Source: CAD feature listing. Evaluate the final solid. Frame: model axes, mm. A direction names the side the tool comes from. Coordinates: 2 decimals unless noted, no trailing zeros. Loops run counter-clockwise (first coordinate to the right, second up) from the corner with the lowest first, then second, coordinate; pieces in that order, holes last. Notation, with made-up numbers: M -10.75,89.5 L 8.25,89.5 A15 cw 8.25,107.5 Z; hole C 17,77.25 d3. An arc over 180 degrees is marked long. One line per question, with ' | ' between items. Start each with the question number.
1. Section query A-A, the plane y = -6.75. Output: boundary loops of the cut face in (x, z), and give its area (3 significant figures).
2. Section query D-D, the plane z = 2.25. Output: boundary loops of the cut face in (x, y).
3. Pin query (flat end, axial travel): P1, Ø6, axis at y = 6, z = -1, coming from the -X side; P2, Ø1.2, axis at x = 143.5, z = -5.5, coming from the +Y side (3 decimals); P3, Ø2, axis at x = 143.5, z = -4.5, coming from the -Y side (3 decimals). Return the tip coordinate at first contact, or that it passes through.
4. Ray query, probe 1 along X at (y, z) = (7.5, -6.5); probe 2 along X at (y, z) = (0.5, -1.25); probe 3 along Y at (x, z) = (3, -4.5). Return the intervals inside material, ascending.
5. Mould query, pull axis X, two halves, no side actions, for faces 1 (the flat face through (-2, -2.375, -5)), 2 (the flat face through (117.25, -4.5, -2.7)), 3 (the flat face through (24.75, 2, 0)), 4 (the flat face through (16.75, -4.5, -2.7)). Classes: pulls with the +X half, pulls with the -X half, needs draft (parallel to the pull), parting line crosses it, or undercut.
6. Section query B-B, the plane z = -4.75. Output: boundary loops of the cut face in (x, y) (3 decimals), and give its area (3 significant figures).
7. Access query for faces 5 (the cylindrical face through (133.508, 4.637, -5.78)), 6 (the flat face through (144, 2.375, -5)), 7 (the flat face through (144, -2.375, -5)), 8 (the cylindrical face through (70.352, 4.637, -5.78)). Directions: +Z, -Z, +X, -X, +Y, -Y. A direction counts if a zero-diameter tool reaches every point of the face in a straight line with its end or side. Return the directions, or none.
8. Section query C-C, the plane y = 0. Output: boundary loops of the cut face in (x, z) (3 decimals).
```python
from build123d import *

# Parameters (mm, degrees)
ESQUISSE5_W        = 4.75
ESQUISSE5_H        = 4.75
BOSS_EXTRU_3_DEPTH = 4
BOSS_EXTRU_4_DEPTH = 4


with BuildPart() as part:
    # Esquisse1 → Révolution1 (revolve)
    with BuildSketch(Plane(origin=(0, 0, 0), x_dir=(1, 0, 0), z_dir=(0, 1, 0))):
        Polygon((0, 0), (0, 4.75), (142, 4.75), (142, 0), (125.25, 0), (125.25, -5), (117.25, -5), (117.25, 0), (24.75, 0), (24.75, -5), (16.75, -5), (16.75, 0), align=None)
    revolve(axis=Axis((0, 0, -4.75), (1, 0, 0)))

    # Esquisse5 → Boss.-Extru.3 (add)
    with BuildSketch(Plane(origin=(142, 0, 0), x_dir=(0, 0, -1), z_dir=(1, 0, 0))):
        with Locations((4.75, 0)):
            Rectangle(ESQUISSE5_W, ESQUISSE5_H)
    extrude(amount=BOSS_EXTRU_3_DEPTH)

    # Esquisse6 → Boss.-Extru.4 (add)
    with BuildSketch(Plane.ZY):
        Polygon((-4.75, 2.375), (-7.125, 2.375), (-7.125, -2.375), (-2.375, -2.375), (-2.375, 2.375), align=None)
    extrude(amount=BOSS_EXTRU_4_DEPTH)


solid = part.part
```
Taken from the geometry:
1) outline: M 16.75,-11.79 L 24.75,-11.79 L 24.75,2.29 L 16.75,2.29 Z; M 117.25,-11.79 L 125.25,-11.79 L 125.25,2.29 L 117.25,2.29 Z | area: 225 mm^2
2) outline: M 16.75,-6.79 L 24.75,-6.79 L 24.75,6.79 L 16.75,6.79 Z; M 117.25,-6.79 L 125.25,-6.79 L 125.25,6.79 L 117.25,6.79 Z
3) P1: x = 0 | P2: y = 2.375 | P3: y = -2.375
4) probe 1: 16.75 to 24.75, 117.25 to 125.25 | probe 2: 0 to 142 | probe 3: -4.74 to 4.74
5) face 1: needs draft | face 2: undercut | face 3: undercut | face 4: pulls with the -X half
6) outline: M -4,-2.375 L 0,-2.375 L 0,-4.75 L 16.75,-4.75 L 16.75,-9.75 L 24.75,-9.75 L 24.75,-4.75 L 117.25,-4.75 L 117.25,-9.75 L 125.25,-9.75 L 125.25,-4.75 L 142,-4.75 L 142,-2.375 L 146,-2.375 L 146,2.375 L 142,2.375 L 142,4.75 L 125.25,4.75 L 125.25,9.75 L 117.25,9.75 L 117.25,4.75 L 24.75,4.75 L 24.75,9.75 L 16.75,9.75 L 16.75,4.75 L 0,4.75 L 0,2.375 L -4,2.375 Z | area: 1,550 mm^2
7) face 5: +X | face 6: +Z, -Z, +X, +Y | face 7: +Z, -Z, +X, -Y | face 8: none
8) outline: M -4,-7.125 L 0,-7.125 L 0,-9.5 L 16.75,-9.5 L 16.75,-14.5 L 24.75,-14.5 L 24.75,-9.5 L 117.25,-9.5 L 117.25,-14.5 L 125.25,-14.5 L 125.25,-9.5 L 142,-9.5 L 142,-7.125 L 146,-7.125 L 146,-2.375 L 142,-2.375 L 142,0 L 125.25,0 L 125.25,5 L 117.25,5 L 117.25,0 L 24.75,0 L 24.75,5 L 16.75,5 L 16.75,0 L 0,0 L 0,-2.375 L -4,-2.375 Z
